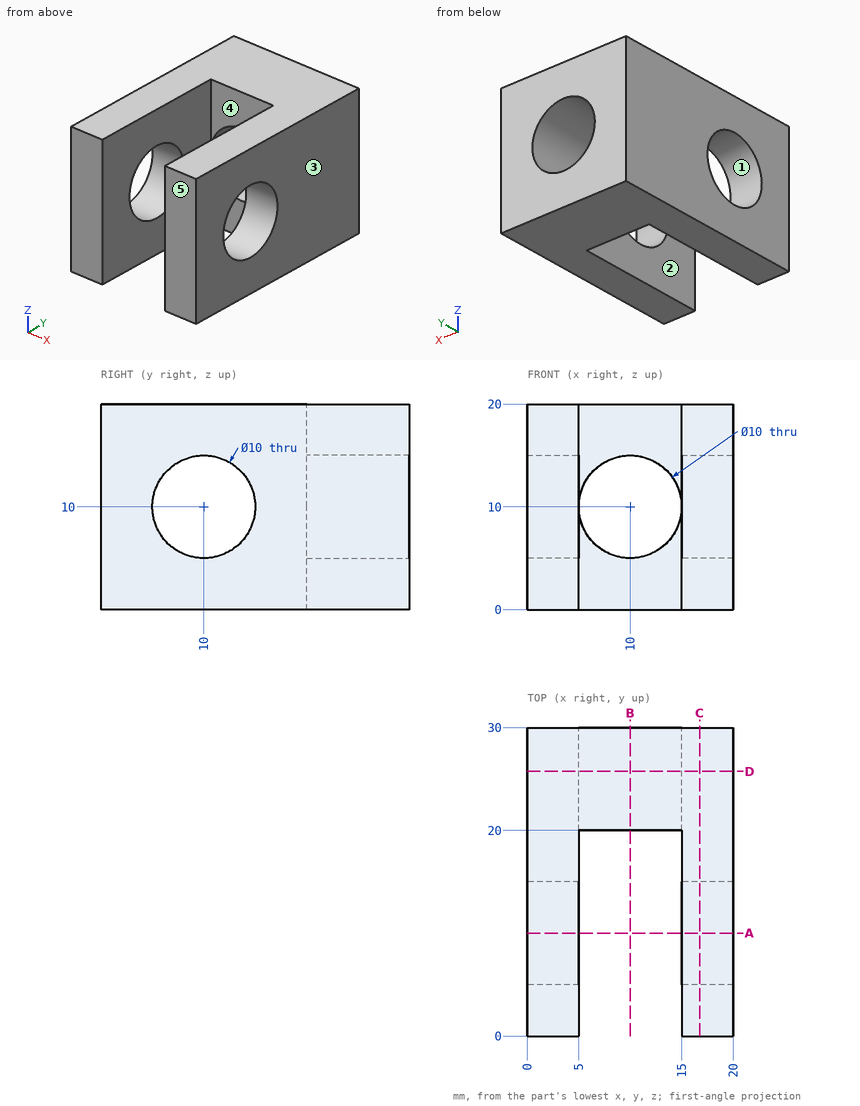
Study the drawing (mm; zero at the part's minimum x, y, z) and answer. A direction names the side the tool comes from. Give positions to 0.01 mm unless a question says otherwise; leave off trailing zeros. Order: outer loops, then holes, each group sorted by start corner. A loop starts at its lowest first (then second) coordinate and runs counter-clockwise, first axis right, second up.
1) Determine the mould class of the marked faces 1, 2 and 3 for opening direction X: pulls with the +X half, pulls with the -X half, needs draft (parallel to the pull), parting line crosses it, or undercut.
Reported:
face 1: needs draft
face 2: undercut
face 3: pulls with the +X half
2) Given P1, Ø11.5, axis at y = 10, z = 10, coming from the +X side; P2, Ø3, axis at x = 9.5, z = 14, coming from the -Y side, each flat-ended and moving along its own axis, determine where each tip first touches the part or whether it passes through.
Reported:
P1: stops at x = 20
P2: stops at y = 20
3) Find section C-C on x = 16.75. Write down the section's boundary in (y, z), then the cut area to 3 significant figures.
Reported:
outline: (0, 0) - (30, 0) - (30, 20) - (0, 20) - close; hole circle Ø10 at (10, 10)
area: 521 mm2
4) Find section B-B on x = 10. Write down the section's boundary in (y, z).
Reported:
outline: (20, 0) - (30, 0) - (30, 5) - (20, 5) - close; (20, 15) - (30, 15) - (30, 20) - (20, 20) - close
5) For the marked faces 4 and 5, determine the directions among +Z, -Z, +X, -X, +Y, -Y from which every point of the face is accessible in a straight line to the end or side of a thin tool.
Reported:
face 4: +Z, -Z, -Y
face 5: +Z, -Z, +X, -X, -Y
6) Find section A-A on y = 10. Write down the section's boundary in (x, z).
Reported:
outline: (0, 0) - (5, 0) - (5, 5) - (0, 5) - close; (0, 15) - (5, 15) - (5, 20) - (0, 20) - close; (15, 0) - (20, 0) - (20, 5) - (15, 5) - close; (15, 15) - (20, 15) - (20, 20) - (15, 20) - close
7) Consider line 1 along X through (y, z) = (18.25, 17.75); line 2 along Y through (x, z) = (17.75, 10). Determine where each line is inside the solid, lowest interval first.
Reported:
line 1: x = 0 to 5, 15 to 20
line 2: y = 0 to 5, 15 to 30
8) Find section D-D on y = 25.75. Write down the section's boundary in (x, z), then the cut area to 3 significant figures.
Reported:
outline: (0, 0) - (20, 0) - (20, 20) - (0, 20) - close; hole circle Ø10 at (10, 10)
area: 321 mm2
